```python
from build123d import *

# Parameters (mm, degrees)
F0_R     = 11.25
F1_DEPTH = 2
F3_DEPTH = 1


with BuildPart() as f1:
    # F0 (on Right) → F1 (new body)
    with BuildSketch(Plane.YZ):
        Circle(F0_R)
    extrude(amount=F1_DEPTH)

    # F2 (on face) → F3 (cut)
    with BuildSketch(Plane(origin=(0, 0, 0), x_dir=(0, -1, 0), z_dir=(-1, 0, 0))):
        with BuildLine():
            Line((-9.75, 0), (-8.25, 0))
            Line((-8.25, 0), (-6.75, 0))
            ThreePointArc((-6.75, 0), (-8.25, 1.5), (-9.75, 0))
        make_face()
        with BuildLine():
            Line((-6.75, 0), (-8.25, 0))
            Line((-8.25, 0), (-9.75, 0))
            ThreePointArc((-9.75, 0), (-8.25, -1.5), (-6.75, 0))
        make_face()
        with BuildLine():
            ThreePointArc((9.75, 0), (8.25, 1.5), (6.75, 0))
            Line((6.75, 0), (8.25, 0))
            Line((8.25, 0), (9.75, 0))
        make_face()
        with BuildLine():
            Line((8.25, 0), (6.75, 0))
            ThreePointArc((6.75, 0), (8.25, -1.5), (9.75, 0))
            Line((9.75, 0), (8.25, 0))
        make_face()
    extrude(amount=-F3_DEPTH, mode=Mode.SUBTRACT)


solid = f1.part
```
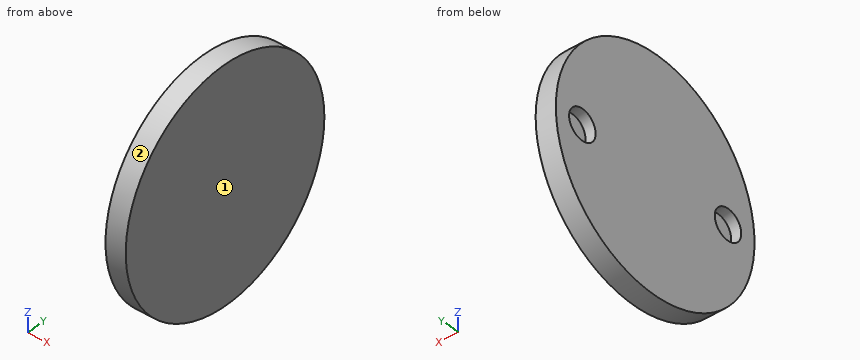
Could you check a few things on this model? Use its own coordinates, in mm. Face numbers are marked on the shaded views. Give positions to 0.01 mm unless a question says otherwise; leave off trailing zeros. Order: outer loops, then holes, each group sorted by start corner. A loop starts at its lowest first (then second) coordinate and runs counter-clockwise, first axis right, second up.
Q1. If I drill on line 1 along Z through (x, y) = (0.5, -8.25); line 2 along Z through (x, y) = (0.75, 8.75); line 3 along Z through (x, y) = (1.8, -2.25), over which ranges is the centre line in solid material (lowest first)?
Q2. We'd pull the mould along Z, two halves only. Please class the marked faces 1 and 2: +Z half, -Z half, draft (parallel to the pull), parting line (faces both ways), or undercut.
Q3. Suppose I cut it at C-C, the plane x = 0.5. Write out the boundary of the cut face in (y, z).
Q4. I'm going to push a flat-ended pin straight in: P1, Ø2.5, axis at y = -8.25, z = 0, coming from the -X side. Where does the tip first touch, or does it pass through?
Q5. Suppose I cut it at A-A, the plane z = 0. Write out the boundary of the cut face in (x, y).
Q6. Suppose I cut it at B-B, the plane y = -8.25. Write out the boundary of the cut face in (x, z).
Q7. Suppose I cut it at D-D, the plane z = 9. Write out the boundary of the cut face in (x, y).
Solution:
1. line 1: z = -7.65 to -1.5, 1.5 to 7.65
1. line 2: z = -7.07 to -1.41, 1.41 to 7.07
1. line 3: z = -11.02 to 11.02
2. face 1: draft
2. face 2: parting line
3. outline: circle Ø22.5 at (0, 0); hole circle Ø3 at (-8.25, 0); hole circle Ø3 at (8.25, 0)
4. P1: stops at x = 1
5. outline: (0, -11.25) - (2, -11.25) - (2, 11.25) - (0, 11.25) - (0, 9.75) - (1, 9.75) - (1, 6.75) - (0, 6.75) - (0, -6.75) - (1, -6.75) - (1, -9.75) - (0, -9.75) - close
6. outline: (0, -7.65) - (2, -7.65) - (2, 7.65) - (0, 7.65) - (0, 1.5) - (1, 1.5) - (1, -1.5) - (0, -1.5) - close
7. outline: (0, -6.75) - (2, -6.75) - (2, 6.75) - (0, 6.75) - close
